Autodesk Fusion 360 part; units mm, degrees
sketch "Sketch1" plane through (0, 0, 0) normal (0, 0, 1) x (1, 0, 0)
  line L0 (-66, -25) -> (66, -25)
  line L1 (66, -25) -> (66.5, 2)
  line L2 (66.5, 2) -> (67.5, 4)
  line L3 (67.5, 4) -> (68, 25)
  line L4 (68, 25) -> (-68, 25)
  line L5 (-68, 25) -> (-67.5, 4)
  line L6 (-67.5, 4) -> (-66.5, 2)
  line L7 (-66.5, 2) -> (-66, -25)
  line L8 (0, 25) -> (0, -25) construction
  line L9 (-66.5, 2) -> (66.5, 2) construction
  line L10 (67.5, 4) -> (-67.5, 4)
  line L11 (-66.5, 2) -> (-64.5, 2)
  line L12 (-64.5, 2) -> (-65, -25)
  line L13 (66.5, 2) -> (64.5, 2)
  line L14 (64.5, 2) -> (65, -25)
  line L15 (-59.5, 25) -> (-59.5, -25)
  line L16 (59.5, 25) -> (59.5, -25)
  point P0 (0, 2)
  point P1 (0, 4)
  dimension "d1" = 132
  dimension "d2" = 133
  dimension "d3" = 27
  dimension "d4" = 29
  dimension "d5" = 50
  dimension "d6" = 136
  dimension "d7" = 135
  dimension "d8" = 1
  dimension "d9" = 2
  dimension "d10" = 1
  dimension "d11" = 2
  dimension "d22" = 8
  dimension "d23" = 8
extrude "Extrude1" add sketch "Sketch1" along normal blind 1.5 contours L0 L7 L11 L12 | L0 L1 L13 L14 makes body 1 at (-66.3333, -7, 0.5) makes body 2 at (64.6667, -7, 0.5)
extrude "Extrude3" add sketch "Sketch1" along normal blind 1 separate body contours L0 L10 L15 L16 | L4 L5 L10 L15 | L4 L10 L15 L16 | L3 L4 L10 L16 makes body 3
extrude "Extrude2" add sketch "Sketch1" against normal blind 1.5 bodies 1 3 2
fillet "Fillet1" radius 1.5 2 edges at (-64.75, -11.5, 1.5) (64.75, -11.5, 1.5) on bodies 1
chamfer "Chamfer1" distance 1 angle 45 2 edges at (0, 25, -1.5) (0, 25, 1) on bodies 1
fillet "Fillet2" radius 1 2 edges at (-65.2752, -25, 0.866) (65.2752, -25, 0.866) on bodies 1
equation "d10 = d8"
equation "d11 = d9"
equation "d23 = d22"
For this review, take the finished solid that the model builds, in its own axes (mm). Coordinates: 2 decimals unless noted, no trailing zeros. Write each loop counter-clockwise with the first axis right and the second up, starting at its lowest first coordinate (ties: lowest second). Pieces come first, ordered by that corner, then holes.
(1) For pin 1 Ø1.5 at (y, z) = (-8, -1) entering from +X; pin 2 Ø6.5 at (x, y) = (-62.5, -4) entering from +Z; pin 3 Ø0.8 at (y, z) = (-17.5, 0.5) entering from +X, all flat-tipped, find the tip position at first contact; note any pin that passes through.
(2) Wall thickness on probe 1 along X at (y, z) = (-5, 0.8); probe 2 along X at (y, z) = (-18.5, 0.3); probe 3 along Z at (x, y) = (-36.5, -19.5): over which ranges is each line inside the solid? List them lowest first.
(3) Add section C-C on y = 21.5. Give the boundary of the cut face in (x, z).
(4) The part is to be moulded in two halves that separate along X. For faces 1 (the face through (-1, 0, 1)), 2 (the face through (-63, -10, 0)), 3 (the face through (-1, 0, -1.5)), say which applies: +X half, -X half, draft (parallel to the pull), parting line (faces both ways), or undercut.
(5) Add section B-B on y = 11.5. Give the boundary of the cut face in (x, z), then the cut area to 3 significant figures.
(6) Add section A-A on x = 28.5. Give the boundary of the cut face in (y, z), then the cut area to 3 significant figures.
Answer sheet:
1. pin 1: stops at x = 66.33
1. pin 2: stops at z = 1.46
1. pin 3: stops at x = 66.15
2. probe 1: x = -66.37 to -64.86, -59.5 to 59.5, 64.86 to 66.37
2. probe 2: x = -66.12 to -64.91, -59.5 to 59.5, 64.91 to 66.12
2. probe 3: z = -1.5 to 1
3. outline: (-67.92, -1.5) - (67.92, -1.5) - (67.92, 1) - (-67.92, 1) - close
4. face 1: undercut
4. face 2: undercut
4. face 3: draft
5. outline: (-67.68, -1.5) - (67.68, -1.5) - (67.68, 1) - (-67.68, 1) - close
5. area: 338 mm2
6. outline: (-25, -1.5) - (24, -1.5) - (25, -0.5) - (25, 0) - (24, 1) - (-25, 1) - close
6. area: 124 mm2
